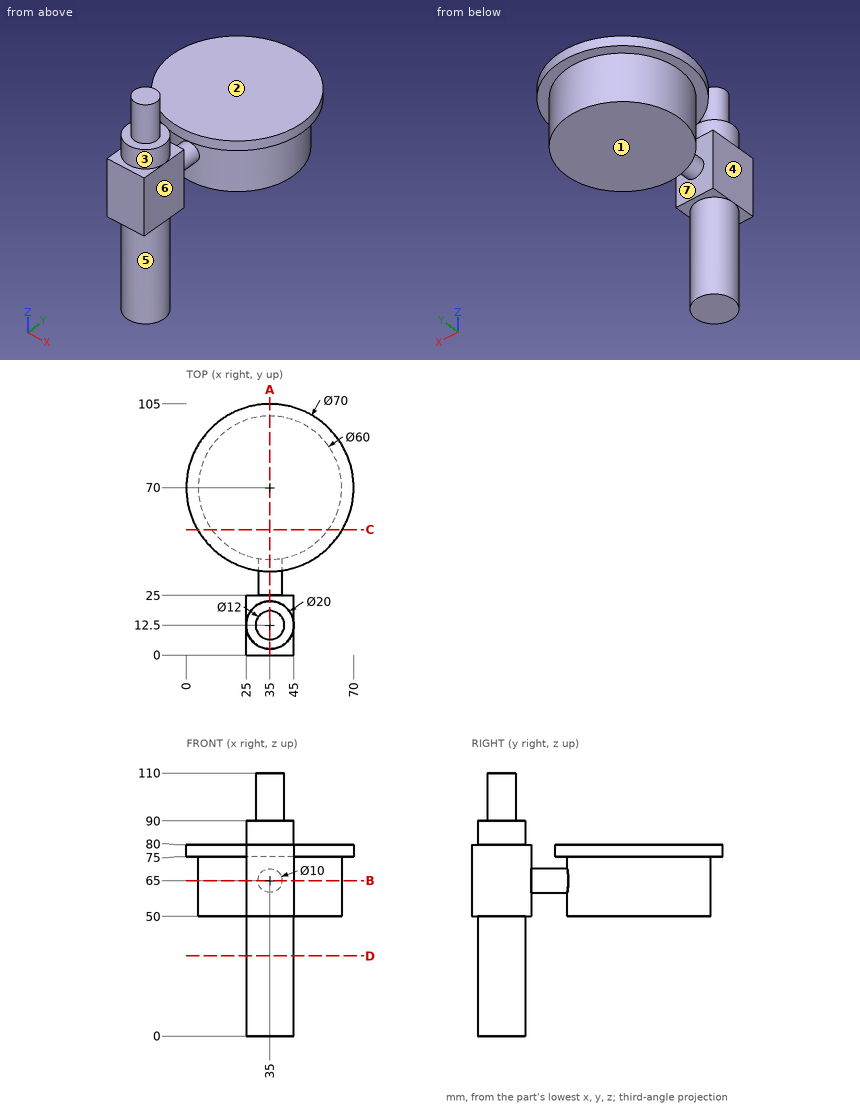
The drawing under review shows one solid part. Ordinate dimensions are in mm from its lowest x, y, z. A direction names the side the tool comes from. Round coordinates to 2 decimals unless told otherwise and drop trailing zeros. Loops run counter-clockwise (first coordinate to the right, second up) from the corner with the lowest first, then second, coordinate; pieces in that order, holes last. Notation, with made-up numbers: M 40.5,67.25 L 99.5,67.25 A22 ccw 99.5,89.25 Z; hole C -3.5,-3.5 d4. An arc over 180 degrees is marked long. Answer as CSV lines item,"result". Start each with the question number.
Item 1: Consider section C-C (y = 52.5). Write out the cut boundary in (x, z), then the cut area to 3 significant figures.
Item 2: For the marked faces 1, 2, 3 and 4, list the 3-axis set-ups (+Z, -Z, +X, -X, +Y, -Y) from which the entire face can be reached by the end or side of a thin tool; tool diameter is ignored.
Item 3: Mouldability with a two-part tool opening along Y and no side actions: class the marked faces 5, 6 and 7 as released by +Y, released by -Y, zero draft, split by the parting line, or undercut.
Item 4: Insertion check: P1, Ø1.5, axis at x = 11.5, z = 62.5, coming from the -Y side; P2, Ø1.5, axis at x = 43, z = 16, coming from the -Y side; P3, Ø5, axis at x = 29.5, z = 31.5, coming from the +Y side. Each pin has a flat end and moves straight along its axis. Give the tip position at first contact, or say it passes through.
Item 5: Consider section D-D (z = 33.5). Write out the cut boundary in (x, y).
Item 6: Consider section A-A (x = 35). Write out the cut boundary in (y, z), then the cut area to 3 significant figures.
Item 7: Wall thickness on line 1 (X direction, y = 10, z = 79); line 2 (Z direction, x = 32, y = 90); line 3 (Z direction, x = 29, y = 19): over which ranges is each line inside the solid? List them lowest first. Write a range as [from, to].
Item 8: Consider section B-B (z = 65). Write out the cut boundary in (x, y), then the cut area to 3 significant figures.
Answer:
1,outline,"M 4.69,75 L 10.63,75 L 10.63,50 L 59.37,50 L 59.37,75 L 65.31,75 L 65.31,80 L 4.69,80 Z"
1,area,"1,520 mm^2"
2,face 1,"-Z, +X, -X, +Y"
2,face 2,"+Z, +X, -X, +Y"
2,face 3,"+Z"
2,face 4,"+Z, -Z, -X, -Y"
3,face 5,"split by the parting line"
3,face 6,"zero draft"
3,face 7,"undercut"
4,P1,"stops at y = 50.44"
4,P2,"stops at y = 5.61"
4,P3,"stops at y = 22.04"
5,outline,"C 35,12.5 d20"
6,outline,"M 0,50 L 2.5,50 L 2.5,0 L 22.5,0 L 22.5,50 L 25,50 L 25,60 L 40,60 L 40,50 L 100,50 L 100,75 L 105,75 L 105,80 L 35,80 L 35,75 L 40,75 L 40,70 L 25,70 L 25,80 L 22.5,80 L 22.5,90 L 18.5,90 L 18.5,110 L 6.5,110 L 6.5,90 L 2.5,90 L 2.5,80 L 0,80 Z"
6,area,"4,190 mm^2"
7,line 1,"x = [25, 45]"
7,line 2,"z = [50, 80]"
7,line 3,"z = [0, 90]"
8,outline,"M 25,0 L 45,0 L 45,25 L 40,25 L 40,40.42 A30 ccw long 30,40.42 L 30,25 L 25,25 Z"
8,area,"3,480 mm^2"
